The model under review builds one solid part; all positions refer to its coordinate system, in mm. A direction names the side the tool comes from. Round coordinates to 2 decimals unless told otherwise and drop trailing zeros. Write each loop counter-clockwise with the first axis right and the second up, starting at its lowest first coordinate (ties: lowest second). Pieces come first, ordered by that corner, then holes. Notation, with made-up numbers: M -9,-28.75 L -1,-28.75 A10 cw -1,-9.75 Z; hole C 88,-20 d8. An arc over 180 degrees is marked long. One line per item, written item: value. Start each with the question number.
1) Wall thickness on probe 1 along Z at (x, y) = (-2, 8.5); probe 2 along Z at (x, y) = (-17, 14.5); probe 3 along X at (y, z) = (57.5, 14.5): over which ranges is each line inside the solid? List them lowest first.
2) Take a section at A-A, the plane z = 4.5. Write out the cut boundary in (x, y).
3) Take a section at B-B, the plane x = -13. Write out the cut boundary in (y, z), and give its area (3 significant figures).
4) Mouldability with a two-part tool opening along X and no side actions: class faces 6 (the face through (4, -3, 26)), 7 (the face through (-12.675, 62.222, 24.958)), 8 (the face through (-12.675, 62.222, 5.916)), 9 (the face through (-12, 59, 22)) as +X half, -X half, draft (parallel to the pull), parting line (faces both ways), or undercut.
5) Take a section at D-D, the plane y = 48.5. Write out the cut boundary in (x, z).
6) Take a section at C-C, the plane z = 15.5. Write out the cut boundary in (x, y).
7) For P1, Ø1.6, axis at x = -19, z = 11, coming from the +Y side; P2, Ø3, axis at x = -11, y = 43.5, coming from the -Z side; P3, Ø5, axis at x = -13, y = 63.69, coming from the +Z side; P4, Ø3, axis at x = -14.5, z = 12.5, coming from the -Y side, all flat-tipped, find the tip position at first contact; note any pin that passes through.
8) Tool access review of faces 1 (the face through (-10.953, 43.692, 6.93)), 2 (the face through (-7.404, 8.695, 25.549)), 3 (the face through (-10, 23, 31)), 4 (the face through (-2.954, 39.474, 29.437)), 5 (the face through (-11.46, 48.69, 25.45)): name each direction out of +Z, -Z, +X, -X, +Y, -Y from which nothing blocks a thin tool from reaching the whole face with its end or side.
from build123d import *

# Parameters (mm, degrees)
F1_DEPTH = 31
F2_W     = 5
F2_H     = 10
F2_H_2   = 20
F3_DEPTH = 25
F5_DEPTH = 31
F6_R     = 1.5
F7_DEPTH = 3


with BuildPart() as f1:
    # F0 (on Top) → F1 (new body)
    with BuildSketch(Plane.XY):
        with BuildLine():
            Line((-18, -5), (0, -5))
            ThreePointArc((0, -5), (3.8729833462, -3.1622776602), (4.8989794856, 1))
            Line((4.8989794856, 1), (-8.1010205144, 64.6867333124))
            ThreePointArc((-8.1010205144, 64.6867333124), (-13.50254481, 68.6614140774), (-18, 63.6867333124))
            ThreePointArc((-18, 63.6867333124), (-17.9640943536, 63.0885968324), (-17.8568931005, 62.4990509432))
            ThreePointArc((-17.8568931005, 62.4990509432), (-17.9284583077, 62.4785593841), (-18, 62.4579858785))
            Line((-18, 62.4579858785), (-18, -5))
        make_face()
        with BuildLine():
            ThreePointArc((-1.5, 0), (0, 1.5), (1.5, 0))
            ThreePointArc((1.5, 0), (1.0606601718, -1.0606601718), (0, -1.5))
            ThreePointArc((0, -1.5), (-1.0606601718, -1.0606601718), (-1.5, 0))
        make_face(mode=Mode.SUBTRACT)
        with BuildLine():
            ThreePointArc((-11.5, 63.6867333124), (-13, 62.1867333124), (-14.5, 63.6867333124))
            ThreePointArc((-14.5, 63.6867333124), (-13, 65.1867333124), (-11.5, 63.6867333124))
        make_face(mode=Mode.SUBTRACT)
    extrude(amount=F1_DEPTH)

    # F2 (on face) → F3 (cut)
    with BuildSketch(Plane(origin=(4.8989794856, 1, 0), x_dir=(-0.2, 0.9797958971, 0), z_dir=(0.9797958971, 0.2, 0))):
        Polygon((0, 22), (0, 2), (45, 2), (45, 12), (65, 12), (65, 22), (50, 22), (50, 29), (10, 29), (10, 22), align=None)
        with Locations((67.5, 17)):
            Rectangle(F2_W, F2_H)
        with Locations((-2.5, 12)):
            Rectangle(F2_W, F2_H_2)
    extrude(amount=-F3_DEPTH, mode=Mode.SUBTRACT)

    # F4 (on face) → F5 (join)
    with BuildSketch(Plane.XY.offset(31)):
        with BuildLine():
            ThreePointArc((-18, 62.4579858785), (-17.9284583077, 62.4785593841), (-17.8568931005, 62.4990509432))
            Line((-17.8568931005, 62.4990509432), (-19.8568931005, 62.4990509432))
            Line((-19.8568931005, 62.4990509432), (-19.8568931005, -5))
            Line((-19.8568931005, -5), (-18, -5))
            Line((-18, -5), (-18, 62.4579858785))
        make_face()
    extrude(amount=-F5_DEPTH)

    # F6 (on face) → F7 (cut)
    with BuildSketch(Plane.XY.offset(31)):
        with BuildLine():
            ThreePointArc((-8, 63.6867333124), (-8.025319235, 64.1892781224), (-8.1010205144, 64.6867333124))
            ThreePointArc((-8.1010205144, 64.6867333124), (-14.0940435791, 68.5655721749), (-17.8568931005, 62.4990509432))
            ThreePointArc((-17.8568931005, 62.4990509432), (-12.40186352, 58.7226389588), (-8, 63.6867333124))
        make_face()
        with Locations((-13, 63.6867333124)):
            Circle(F6_R, mode=Mode.SUBTRACT)
    extrude(amount=-F7_DEPTH, mode=Mode.SUBTRACT)


solid = f1.part
Checked values:
1. probe 1: z = 0 to 2, 22 to 31
1. probe 2: z = 0 to 2, 29 to 31
1. probe 3: x = -19.86 to -18
2. outline: M -19.86,-5 L -18,-5 L -18,42.25 L -4.1,45.09 L -8.1,64.69 A5 ccw long -17.86,62.5 L -19.86,62.5 Z; hole C -13,63.69 d3
3. outline: M -5,0 L 62.19,0 L 62.19,12 L 43.27,12 L 43.27,2 L -5,2 Z; M -5,22 L 7.55,22 L 7.55,29 L 48.38,29 L 48.38,22 L 62.19,22 L 62.19,28 L 58.69,28 L 58.69,31 L -5,31 Z; M 65.19,0 L 68.69,0 L 68.69,12 L 65.19,12 Z; M 65.19,22 L 68.69,22 L 68.69,28 L 65.19,28 Z
3. area: 695 mm2
4. face 6: +X half
4. face 7: undercut
4. face 8: undercut
4. face 9: draft
5. outline: M -19.86,0 L -4.8,0 L -4.8,12 L -18,12 L -18,22 L -12.4,22 L -12.4,29 L -4.8,29 L -4.8,31 L -19.86,31 Z
6. outline: M -19.86,-5 L -18,-5 L -18,62.46 A65 cw -17.86,62.5 L -19.86,62.5 Z
7. P1: stops at y = 62.5
7. P2: stops at z = 0
7. P3: stops at z = 28
7. P4: stops at y = 42.68
8. face 1: +X, -Y
8. face 2: none
8. face 3: +Z, +X, -X, +Y, -Y
8. face 4: +Z, -Z, +X, +Y
8. face 5: +X
